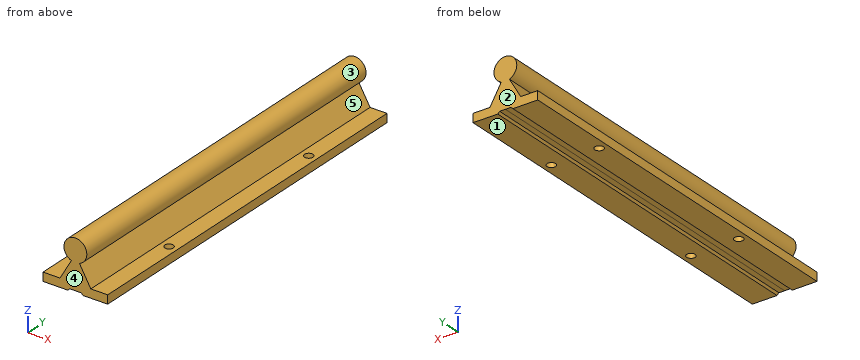
from build123d import *

# Parameters (mm, degrees)
F1_DEPTH = 200
F2_R     = 6
F3_DEPTH = 200
F4_R     = 2.25
F5_DEPTH = 26.461


with BuildPart() as f1:
    # F0 (on Front) → F1 (new body)
    with BuildSketch(Plane.XZ):
        with BuildLine():
            ThreePointArc((2.153722, 13.845509), (1.107413, 13.556125), (0.026086, 13.460011))
            ThreePointArc((0.026086, 13.460011), (-1.054859, 13.560315), (-2.100039, 13.853753))
            Line((-2.100039, 13.853753), (-8.086373, 3.53137))
            Line((-8.086373, 3.53137), (-16.986306, 3.565868))
            Line((-16.986306, 3.565868), (-17.003748, -0.934098))
            Line((-17.003748, -0.934098), (-4.003846, -0.984488))
            Line((-4.003846, -0.984488), (-2.999977, 0.011628))
            Line((-2.999977, 0.011628), (0, 0))
            Line((0, 0), (3, 0))
            Line((3, 0), (4, -1))
            Line((4, -1), (17, -1))
            Line((17, -1), (17, 3.5))
            Line((17, 3.5), (8.1, 3.5))
            Line((8.1, 3.5), (2.153722, 13.845509))
        make_face()
    extrude(amount=-F1_DEPTH)

    # F2 (on Front) → F3 (join)
    with BuildSketch(Plane.XZ):
        with Locations((0, 19.46)):
            Circle(F2_R)
    extrude(amount=-F3_DEPTH)

    # F4 (on face) → F5 (cut, through all)
    with BuildSketch(Plane(origin=(0, 0, -1), x_dir=(1, 0, 0), z_dir=(0, 0, -1))):
        with Locations((12.55, -50)):
            Circle(F4_R)
        with Locations((12.55, -150)):
            Circle(F4_R)
        with Locations((-12.55, -150)):
            Circle(F4_R)
        with Locations((-12.55, -50)):
            Circle(F4_R)
    extrude(amount=-F5_DEPTH, mode=Mode.SUBTRACT)


solid = f1.part
Verification items for the finished model (mm, model axes). Face numbers are marked on the shaded views. A direction names the side the tool comes from. Give positions to 0.01 mm unless a question says otherwise; leave off trailing zeros. Write each loop counter-clockwise with the first axis right and the second up, starting at its lowest first coordinate (ties: lowest second). Pieces come first, ordered by that corner, then holes. Notation, with made-up numbers: M 73.5,-17.5 L 105.5,-17.5 A21 ccw 105.5,16.5 Z; hole C 87.25,-28 d5. An arc over 180 degrees is marked long. Put each result on its own line as item: value. Start each with the question number.
1. Section check B-B (y = 150). Give the number of separate pieces and of enclosed holes in the cut face, and give its area (3 significant figures).
2. Section check D-D (x = -12.55). Record the cut outline in (y, z), and give its area (3 significant figures).
3. Section check A-A (x = 12.55). Record the cut outline in (y, z).
4. Scan lines: line 1 along Y through (x, z) = (12.55, 0.5); line 2 along X through (y, z) = (150, 1.45); line 3 along Z through (x, y) = (-10.5, 31). Record each from-to range of solid material in increasing order. Write a range as [from, to].
5. Go/stop test with flat-tipped pins: pin 1 Ø10 at (y, z) = (73, 7) entering from -X; pin 2 Ø6 at (x, y) = (2.5, 23.5) entering from +Z; pin 3 Ø8 at (x, y) = (-4, 103.5) entering from -Z; pin 4 Ø2 at (x, y) = (-8.5, 161.5) entering from +Z. Record where each tip stops, or that it passes through.
6. Set-up check for the marked faces 4 and 5: record each of +Z, -Z, +X, -X, +Y, -Y from which the full face is reachable in a straight line by a thin tool's end or side.
7. Draft check along Z on the marked faces 1, 2 and 3. Enter one of: +Z half, -Z half, draft (parallel to the pull), parting line (faces both ways), or undercut.
Answer list:
1. separate pieces: 3
1. enclosed holes: 0
1. area: 323 mm2
2. outline: M 0,-0.95 L 47.75,-0.95 L 47.75,3.55 L 0,3.55 Z; M 52.25,-0.95 L 147.75,-0.95 L 147.75,3.55 L 52.25,3.55 Z; M 152.25,-0.95 L 200,-0.95 L 200,3.55 L 152.25,3.55 Z
2. area: 860 mm2
3. outline: M 0,-1 L 47.75,-1 L 47.75,3.5 L 0,3.5 Z; M 52.25,-1 L 147.75,-1 L 147.75,3.5 L 52.25,3.5 Z; M 152.25,-1 L 200,-1 L 200,3.5 L 152.25,3.5 Z
4. line 1: [0, 47.75], [52.25, 147.75], [152.25, 200]
4. line 2: [-16.99, -14.8], [-10.3, 10.3], [14.8, 17]
4. line 3: [-0.96, 3.54]
5. pin 1: x = -16.99
5. pin 2: z = 25.46
5. pin 3: z = -0.98
5. pin 4: z = 4.54
6. face 4: +Z, -Z, +X, -X, -Y
6. face 5: +X, +Y, -Y
7. face 1: -Z half
7. face 2: draft
7. face 3: undercut
